Part model, mm, in its own coordinate system. A direction names the side the tool comes from. Round coordinates to 2 decimals unless told otherwise and drop trailing zeros. Order: outer loops, then holes, each group sorted by start corner. A loop starts at its lowest first (then second) coordinate and runs counter-clockwise, first axis right, second up. Notation, with made-up numbers: (56.25, -14.5) - (91.25, -14.5) arc R30 cw to (91.25, 15.5) - close; hole circle Ø8 at (-14, 64.5). An arc over 180 degrees is marked (long way). Answer as a JSON object with one key per item and string values.
```python
from build123d import *

# Parameters (mm, degrees)
F0_R     = 20
F1_DEPTH = 15
F2_R     = 18
F3_DEPTH = 13
F5_R     = 3.5
F5_R_2   = 1.5
F6_DEPTH = 16
F8_DEPTH = 2


with BuildPart() as f1:
    # F0 (on Top) → F1 (new body)
    with BuildSketch(Plane.XY):
        Circle(F0_R)
    extrude(amount=F1_DEPTH)

    # F2 (on face) → F3 (cut)
    with BuildSketch(Plane.XY.offset(15)):
        Circle(F2_R)
    extrude(amount=-F3_DEPTH, mode=Mode.SUBTRACT)

    # F5 (on face) → F6 (join)
    with BuildSketch(Plane.XY.offset(2)):
        Circle(F5_R)
        Circle(F5_R_2, mode=Mode.SUBTRACT)
    extrude(amount=F6_DEPTH)

    # F7 (on face) → F8 (cut)
    with BuildSketch(Plane.XY.offset(2)):
        with BuildLine():
            Line((-3.8471836237, -3.068026562), (-17.26724866, -5.0835148974))
            ThreePointArc((-17.26724866, -5.0835148974), (-14.0729666844, -11.2228164335), (-8.7983848642, -15.7031342025))
            Line((-8.7983848642, -15.7031342025), (-3.8471836237, -3.068026562))
        make_face()
        with BuildLine():
            Line((0, -4.9207325491), (-6.7915014573, -16.6695983142))
            ThreePointArc((-6.7915014573, -16.6695983142), (0, -18), (6.7915014573, -16.6695983142))
            Line((6.7915014573, -16.6695983142), (0, -4.9207325491))
        make_face()
        with BuildLine():
            Line((-4.7973595105, 1.0949660026), (-14.7404054341, 10.3305589219))
            ThreePointArc((-14.7404054341, 10.3305589219), (-17.5487024193, 4.0053768112), (-17.7629079286, -2.9118897508))
            Line((-17.7629079286, -2.9118897508), (-4.7973595105, 1.0949660026))
        make_face()
        with BuildLine():
            Line((-2.1350258376, 4.433426834), (-1.1137362668, 17.965511168))
            ThreePointArc((-1.1137362668, 17.965511168), (-7.8099073041, 16.2174396222), (-13.3515990255, 12.072067075))
            Line((-13.3515990255, 12.072067075), (-2.1350258376, 4.433426834))
        make_face()
        with BuildLine():
            ThreePointArc((13.3515990255, 12.072067075), (7.8099073041, 16.2174396222), (1.1137362668, 17.965511168))
            Line((1.1137362668, 17.965511168), (2.1350258376, 4.433426834))
            Line((2.1350258376, 4.433426834), (13.3515990255, 12.072067075))
        make_face()
        with BuildLine():
            ThreePointArc((18, 0), (17.1657696858, 5.4163041913), (14.7404054341, 10.3305589219))
            Line((14.7404054341, 10.3305589219), (4.7973595105, 1.0949660026))
            Line((4.7973595105, 1.0949660026), (17.7629079286, -2.9118897508))
            ThreePointArc((17.7629079286, -2.9118897508), (17.940629068, -1.4607630344), (18, 0))
        make_face()
        with BuildLine():
            ThreePointArc((8.7983848642, -15.7031342025), (14.0729666844, -11.2228164335), (17.26724866, -5.0835148974))
            Line((17.26724866, -5.0835148974), (3.8471836237, -3.068026562))
            Line((3.8471836237, -3.068026562), (8.7983848642, -15.7031342025))
        make_face()
    extrude(amount=-F8_DEPTH, mode=Mode.SUBTRACT)


solid = f1.part
```
Item 1: Two-plate mould, pull along Y, no slides. Class faces 1 (the flat face through (-18, 3, 15)), 2 (the cylindrical face through (-4.336, -19.524, 7.395)), 3 (the flat face through (6.29, -9.3, 1.01)), 4 (the cylindrical face through (-1.5, 0.07, 9.89)): pulls with the +Y half, pulls with the -Y half, needs draft (parallel to the pull), parting line crosses it, or undercut.
Taken from the geometry:
{"face 1": "needs draft", "face 2": "parting line crosses it", "face 3": "undercut", "face 4": "undercut"}
Item 2: Cut at A-A (z = 11.25). Write the cut outline in (x, y).
Taken from the geometry:
{"outline": "circle Ø40 at (0, 0); circle Ø7 at (0, 0); hole circle Ø36 at (0, 0); hole circle Ø3 at (0, 0)"}
Item 3: Cut at C-C (y = 5.5). Write the cut outline in (x, z).
Taken from the geometry:
{"outline": "(-19.23, 0) - (-17.14, 0) - (-17.14, 15) - (-19.23, 15) - close; (-9.54, 0) - (-3.7, 0) - (-3.7, 2) - (-9.54, 2) - close; (-2.05, 0) - (2.05, 0) - (2.05, 2) - (-2.05, 2) - close; (3.7, 0) - (9.54, 0) - (9.54, 2) - (3.7, 2) - close; (17.14, 0) - (19.23, 0) - (19.23, 15) - (17.14, 15) - close"}
Item 4: Cut at D-D (x = 5.5). Write the cut outline in (y, z).
Taken from the geometry:
{"outline": "(-19.23, 0) - (-17.14, 0) - (-17.14, 15) - (-19.23, 15) - close; (-14.44, 0) - (-7.29, 0) - (-7.29, 2) - (-14.44, 2) - close; (-3.32, 0) - (0.88, 0) - (0.88, 2) - (-3.32, 2) - close; (1.75, 0) - (6.73, 0) - (6.73, 2) - (1.75, 2) - close; (17.14, 0) - (19.23, 0) - (19.23, 15) - (17.14, 15) - close"}
Item 5: Drop flat-ended pins along their axis: P1, Ø8, axis at x = -12, y = 4, coming from the -Z side; P2, Ø3, axis at x = 9, z = 9, coming from the +Y side; P3, Ø10, axis at x = 9.5, z = 5, coming from the +Y side; P4, Ø0.9, axis at x = 0.5, y = 0.5, coming from the +Z side. Give the stop position or say it passes through.
Taken from the geometry:
{"P1": "z = 0", "P2": "y = 18.54", "P3": "y = 19.49", "P4": "z = 2"}
Item 6: Tool access for faces 5 (the flat face through (-3.348, -10.713, 1.014)), 6 (the cylindrical face through (3.233, -1.341, 9.888)), 7 (the flat face through (0, -2, 18)): list every direction of +Z, -Z, +X, -X, +Y, -Y with a clear straight run to the whole face (end or side of a thin tool).
Taken from the geometry:
{"face 5": "+Z, -Z", "face 6": "+Z", "face 7": "+Z, +X, -X, +Y, -Y"}
Item 7: Probe L1, parallel to Y at x = 0, z = 13.5; L2, parallel to Y at x = 2, z = 8; L3, parallel to X at y = -2.5, z = 7. List the from-to ranges inside material, lowest first. Write a range as from..to.
Taken from the geometry:
{"L1": "-20..-18, -3.5..-1.5, 1.5..3.5, 18..20", "L2": "-19.9..-17.89, -2.87..2.87, 17.89..19.9", "L3": "-19.84..-17.83, -2.45..2.45, 17.83..19.84"}
Item 8: Cut at B-B (y = -7.5). Write the cut outline in (x, z), plus the area to 3 significant figures.
Taken from the geometry:
{"outline": "(-18.54, 0) - (-16.36, 0) - (-16.36, 15) - (-18.54, 15) - close; (-5.58, 0) - (-1.49, 0) - (-1.49, 2) - (-5.58, 2) - close; (1.49, 0) - (5.58, 0) - (5.58, 2) - (1.49, 2) - close; (16.36, 0) - (18.54, 0) - (18.54, 15) - (16.36, 15) - close", "area": "81.7 mm2"}
